```python
from build123d import *

# Parameters (mm, degrees)
F0_R     = 42
F0_R_2   = 13
F3_DEPTH = 21
F4_DEPTH = 25
F9_DEPTH = 18


# Not quite as in the source:
# - a feature names something its author has since deleted; it is built from what else it names


with BuildPart() as f3:
    # F0 (on Top) → F3 (new body)
    with BuildSketch(Plane.XY):
        Circle(F0_R)
        Circle(F0_R_2, mode=Mode.SUBTRACT)
    extrude(amount=F3_DEPTH)

    # F2 (on offset) → F4 (cut)
    with BuildSketch(Plane.XY.offset(2)):
        with BuildLine():
            Line((1, 43.9886348958), (1, 14.9666295471))
            ThreePointArc((1, 14.9666295471), (6.5082560868, 13.5145330185), (11.0778923645, 10.1133723733))
            Line((11.0778923645, 10.1133723733), (33.7682098305, 28.2082967377))
            ThreePointArc((33.7682098305, 28.2082967377), (19.0908845212, 39.6426301877), (1, 43.9886348958))
        make_face()
        with BuildLine():
            ThreePointArc((-11.0778923645, 10.1133723733), (-6.5082560868, 13.5145330185), (-1, 14.9666295471))
            Line((-1, 14.9666295471), (-1, 43.9886348958))
            ThreePointArc((-1, 43.9886348958), (-19.0908845212, 39.6426301877), (-33.7682098305, 28.2082967377))
            Line((-33.7682098305, 28.2082967377), (-11.0778923645, 10.1133723733))
        make_face()
        with BuildLine():
            ThreePointArc((-7.3947460578, -13.0505835402), (-11.727472237, -9.3523470279), (-14.3688639628, -4.3053162972))
            Line((-14.3688639628, -4.3053162972), (-42.6632270448, -10.7633200327))
            ThreePointArc((-42.6632270448, -10.7633200327), (-34.4005852286, -27.4335512818), (-19.9869222552, -39.1985068436))
            Line((-19.9869222552, -39.1985068436), (-7.3947460578, -13.0505835402))
        make_face()
        with BuildLine():
            ThreePointArc((5.592808322, -13.9183510185), (0, -15), (-5.592808322, -13.9183510185))
            Line((-5.592808322, -13.9183510185), (-18.1849845194, -40.0662743218))
            ThreePointArc((-18.1849845194, -40.0662743218), (0, -44), (18.1849845194, -40.0662743218))
            Line((18.1849845194, -40.0662743218), (5.592808322, -13.9183510185))
        make_face()
        with BuildLine():
            ThreePointArc((14.3688639628, -4.3053162972), (11.727472237, -9.3523470279), (7.3947460578, -13.0505835402))
            Line((7.3947460578, -13.0505835402), (19.9869222552, -39.1985068436))
            ThreePointArc((19.9869222552, -39.1985068436), (34.4005852286, -27.4335512818), (42.6632270448, -10.7633200327))
            Line((42.6632270448, -10.7633200327), (14.3688639628, -4.3053162972))
        make_face()
        with BuildLine():
            ThreePointArc((12.3248719682, 8.5497094083), (14.6239186827, 3.3378140093), (14.8139058307, -2.3554604728))
            Line((14.8139058307, -2.3554604728), (43.1082689127, -8.8134642083))
            ThreePointArc((43.1082689127, -8.8134642083), (42.896828136, 9.7909210941), (35.0151894342, 26.6446337728))
            Line((35.0151894342, 26.6446337728), (12.3248719682, 8.5497094083))
        make_face()
    extrude(amount=F4_DEPTH, mode=Mode.SUBTRACT)

    # F8 (on offset) → F9 (cut)
    with BuildSketch(Plane.XY):
        with BuildLine():
            Line((-39.2080294912, -7.9232600118), (-12.8590309309, -1.9092730337))
            ThreePointArc((-12.8590309309, -1.9092730337), (-12.6740628584, 2.8927721414), (-10.7571840173, 7.2995199854))
            Line((-10.7571840173, 7.2995199854), (-31.8874402635, 24.150337042))
            ThreePointArc((-31.8874402635, 24.150337042), (-38.9976968795, 8.900969829), (-39.2080294912, -7.9232600118))
        make_face()
    extrude(amount=F9_DEPTH, mode=Mode.SUBTRACT)


solid = f3.part
```
Build history of the part. All positions in model axes, mm. A direction names the side the tool comes from. Coordinates: 2 decimals unless noted, no trailing zeros. Order: outer loops, then holes, each group sorted by start corner. A loop starts at its lowest first (then second) coordinate and runs counter-clockwise, first axis right, second up. Notation, with made-up numbers: (-40, 1.5) -> (-25, 1.5) arc R22 ccw to (-25, 17.5) -> close; hole circle Ø5 at (75.25, 34.5). An arc over 180 degrees is marked (long way). Answer in a Markdown table with one row per item. Add a question column.
Q1. Which spindle directions (+Z, -Z, +X, -X, +Y, -Y) get a long thin tool onto all of the face, cutting with end or side? Do faces 4 (the face through (12, -9, 11)), 5 (the face through (-6.58, 13.48, 11.37)), 6 (the face through (23.036, 17.091, 11.367)), 7 (the face through (-29, 5, 18)). Say none if no direction does.
Q2. Mould opens along Y. For faces 1 (the face through (0, -15, 11)), 2 (the face through (21.493, 18.419, 11.367)), 3 (the face through (27.8, -5.32, 11.37)) say: +Y half, -Y half, draft (parallel to the pull), parting line (faces both ways), or undercut.
Q3. Wall check: line 1 along X through (y, z) = (0, 8.5); line 2 along X through (y, z) = (18, 15.25); line 3 along X through (y, z) = (22, 6.75). Give the ranges that are in metal, low to high. Write a range as [from, to].
Q4. Band-saw the part on A-A, the plane y = 0. List the corners of the cut face in (x, z).
Q5. Drop flat-ended pins along their axis: pin 1 (8.5 mm diameter, centred on x = -3.5, y = -29, fed in from +Z); pin 2 (1 mm diameter, centred on x = 17, z = 12, fed in from -Y); pin 3 (2 mm diameter, centred on y = 31.5, z = 10, fed in from +X); pin 4 (2 mm diameter, centred on x = -8.5, y = -7.5, fed in from +Z). Give the stop position or say it passes through.
Q6. Band-saw the part on C-C, the plane z = 10.5. List the corners of the cut face in (x, y).
Q7. Band-saw the part on D-D, the plane x = -16. List the corners of the cut face in (y, z), then the cut area to 3 significant figures.
Q8. Band-saw the part on B-B, the plane x = 0. List the corners of the cut face in (y, z), then the cut area to 3 significant figures.
Answers follow:
| question | item | result |
|---|---|---|
| 1 | face 4 | +Z |
| 1 | face 5 | +Z, +Y |
| 1 | face 6 | +Z, +X |
| 1 | face 7 | -Z |
| 2 | face 1 | -Y half |
| 2 | face 2 | +Y half |
| 2 | face 3 | undercut |
| 3 | line 1 | [-42, -40], [13, 15] |
| 3 | line 2 | [-37.95, -35.72], [-24.18, -20.97], [-1, 1], [20.97, 24.18] |
| 3 | line 3 | [-35.78, -33.41], [-29.19, -25.98], [-1, 1], [25.98, 29.19] |
| 4 | outline | (-42, 0) -> (-40, 0) -> (-40, 18) -> (-13, 18) -> (-13, 21) -> (-42, 21) -> close; (13, 0) -> (42, 0) -> (42, 2) -> (15, 2) -> (15, 21) -> (13, 21) -> close |
| 5 | pin 1 | z = 2 |
| 5 | pin 2 | y = -38.26 |
| 5 | pin 3 | x = 1 |
| 5 | pin 4 | through |
| 6 | outline | (-40.71, -10.32) -> (-14.37, -4.31) arc R15 ccw to (-7.39, -13.05) -> (-19.12, -37.4) arc R42 ccw to (-17.32, -38.26) -> (-5.59, -13.92) arc R15 ccw to (5.59, -13.92) -> (17.32, -38.26) arc R42 ccw to (19.12, -37.4) -> (7.39, -13.05) arc R15 ccw to (14.37, -4.31) -> (40.71, -10.32) arc R42 ccw to (41.16, -8.37) -> (14.81, -2.36) arc R15 ccw to (12.32, 8.55) -> (33.45, 25.4) arc R42 ccw to (32.2, 26.96) -> (11.08, 10.11) arc R15 ccw to (1, 14.97) -> (1, 41.99) arc R42 ccw to (-1, 41.99) -> (-1, 14.97) arc R15 ccw to (-11.08, 10.11) -> (-32.2, 26.96) arc R42 ccw to start; hole (-39.21, -7.92) -> (-12.86, -1.91) arc R13 ccw (long way) to (-10.76, 7.3) -> (-31.89, 24.15) arc R40 ccw to start |
| 7 | outline | (-38.83, 0) -> (-2.63, 0) -> (-2.63, 18) -> (11.48, 18) -> (11.48, 0) -> (38.83, 0) -> (38.83, 2) -> (14.04, 2) -> (14.04, 21) -> (-4.68, 21) -> (-4.68, 2) -> (-30.92, 2) -> (-30.92, 21) -> (-35.53, 21) -> (-35.53, 2) -> (-38.83, 2) -> close |
| 7 | area | 345 mm^2 |
| 8 | outline | (-42, 0) -> (-13, 0) -> (-13, 21) -> (-15, 21) -> (-15, 2) -> (-42, 2) -> close; (13, 0) -> (42, 0) -> (42, 21) -> (13, 21) -> close |
| 8 | area | 705 mm^2 |
